For this review, take the finished solid that the model builds, in its own axes (mm). A direction names the side the tool comes from. Give positions to 0.01 mm unless a question says otherwise; leave off trailing zeros. Loops run counter-clockwise (first coordinate to the right, second up) from the corner with the lowest first, then second, coordinate; pieces in that order, holes last.
```python
from build123d import *

# Parameters (mm, degrees)
SKETCH1_W                  = 12.065
SKETCH1_H                  = 15.875
BASE_DEPTH                 = 15.875
SKETCH3_R                  = 1.397
SHAFTHOLE_DEPTH            = 19.745948562
SKETCH7_W                  = 18.144441676
SKETCH7_H                  = 22.667604572
SKETCH7_W_2                = 6.35
SKETCH7_H_2                = 10.16
CUT_EXTRUDE1_DEPTH         = 10.795
F_4_40_TAPPED_HOLE1_REACH  = 27.692
F_4_40_TAPPED_HOLE1_BORE_R = 1.1303


with BuildPart() as part:
    # Sketch1 → Base (new body)
    with BuildSketch(Plane.XY):
        Rectangle(SKETCH1_W, SKETCH1_H)
    extrude(amount=BASE_DEPTH)

    # Sketch3 → ShaftHole (cut, through all)
    with BuildSketch(Plane(origin=(0, 0, 0), x_dir=(-1, 0, 0), z_dir=(0, 0, -1))):
        with Locations((0, 3.1877)):
            Circle(SKETCH3_R)
    extrude(amount=-SHAFTHOLE_DEPTH, mode=Mode.SUBTRACT)

    # Sketch7 → Cut-Extrude1 (cut)
    with BuildSketch(Plane(origin=(0, 7.9375, 0), x_dir=(1, 0, 0), z_dir=(0, 1, 0))):
        with Locations((0.669483701, -7.615912702)):
            Rectangle(SKETCH7_W, SKETCH7_H)
        with Locations((0, -5.08)):
            Rectangle(SKETCH7_W_2, SKETCH7_H_2, mode=Mode.SUBTRACT)
    extrude(amount=-CUT_EXTRUDE1_DEPTH, mode=Mode.SUBTRACT)

    # #4-40 Tapped Hole1 bore → #4-40 Tapped Hole1 (cut, up to next)
    with BuildSketch(Plane(origin=(5.103236707, 7.9375, -0.979692924), x_dir=(0, 0, 1), z_dir=(0, 1, 0)), mode=Mode.PRIVATE) as f_4_40_tapped_hole1_sk1:
        with Locations((6.059692924, -5.103236707)):
            Circle(F_4_40_TAPPED_HOLE1_BORE_R)
    f_4_40_tapped_hole1_tool1 = extrude(f_4_40_tapped_hole1_sk1.sketch, amount=-F_4_40_TAPPED_HOLE1_REACH, mode=Mode.PRIVATE) & part.part
    add(f_4_40_tapped_hole1_tool1.solids().sort_by_distance((0, 7.9375, 5.08))[0], mode=Mode.SUBTRACT)


solid = part.part
```
Item 1: Take a section at C-C on z = 5.08. Give the boundary of the cut face in (x, y) (1 decimal).
Answer:
outline: (-6, -7.9) - (6, -7.9) - (6, -2.9) - (3.2, -2.9) - (3.2, 7.9) - (1.1, 7.9) - (1.1, 4) arc R1.4 cw (long way) to (-1.1, 4) - (-1.1, 7.9) - (-3.2, 7.9) - (-3.2, -2.9) - (-6, -2.9) - close
Item 2: For L1, parallel to Z at x = 0, y = 6.9; L2, parallel to Y at x = 0, z = 7; L3, parallel to X at y = 5, z = 5.08 (3 decimals), list the stretches that pass through material, from the lowest coordinate up.
Answer:
L1: z = 0 to 3.95, 6.21 to 10.16
L2: y = -7.94 to 1.79, 4.58 to 7.94
L3: x = -3.175 to -1.13, 1.13 to 3.175
Item 3: Take a section at D-D on z = 8. Give the boundary of the cut face in (x, y) (1 decimal), and give its area (3 significant figures).
Answer:
outline: (-6, -7.9) - (6, -7.9) - (6, -2.9) - (3.2, -2.9) - (3.2, 7.9) - (-3.2, 7.9) - (-3.2, -2.9) - (-6, -2.9) - close; hole circle Ø2.8 at (0, 3.2)
area: 124 mm2
Item 4: Clearance check with flat-ended pins moving along their axes: pin 1 Ø7 at (x, y) = (-1, 0) entering from +Z (3 decimals); pin 2 Ø6 at (y, z) = (2.5, 2.5) entering from -X (3 decimals); pin 3 Ø8 at (y, z) = (4.5, 3.5) entering from +X (3 decimals). State where each tip first meets the part, or that it passes through.
Answer:
pin 1: stops at z = 15.875
pin 2: stops at x = -3.175
pin 3: stops at x = 3.175
Item 5: Tool access review of faces 5 (the flat face through (0, 1, 10.16)), 6 (the flat face through (3.175, 3, 5)), 7 (the flat face through (1, 7.938, 4)), 8 (the flat face through (-3.175, 3, 5)): name each direction out of +Z, -Z, +X, -X, +Y, -Y from which nothing blocks a thin tool from reaching the whole face with its end or side.
Answer:
face 5: +Z, +X, -X, +Y
face 6: +Z, -Z, +X, +Y
face 7: +Z, -Z, +X, -X, +Y
face 8: +Z, -Z, -X, +Y
Item 6: Take a section at B-B on x = 0. Give the boundary of the cut face in (y, z) (1 decimal), and give its area (3 significant figures).
Answer:
outline: (-7.9, 0) - (1.8, 0) - (1.8, 10.2) - (-2.9, 10.2) - (-2.9, 15.9) - (-7.9, 15.9) - close; (4.6, 0) - (7.9, 0) - (7.9, 3.9) - (4.6, 3.9) - close; (4.6, 6.2) - (7.9, 6.2) - (7.9, 10.2) - (4.6, 10.2) - close
area: 154 mm2
Item 7: Take a section at A-A on y = 3.5. Give the boundary of the cut face in (x, z) (3 decimals), and give its area (3 significant figures).
Answer:
outline: (-3.175, 0) - (-1.362, 0) - (-1.362, 10.16) - (-3.175, 10.16) - close; (1.362, 0) - (3.175, 0) - (3.175, 10.16) - (1.362, 10.16) - close
area: 36.8 mm2
Item 8: The part is to be moulded in two halves that separate along X. For faces 1 (the flat face through (-6.032, -5, 8)), 2 (the flat face through (0, -2, 0)), 3 (the cylindrical face through (0.34, 6, 6.16)), 4 (the cylindrical face through (0.303, 1.824, 5.009)), say which applies: released by +X, released by -X, zero draft, split by the parting line, or undercut.
Answer:
face 1: released by -X
face 2: zero draft
face 3: undercut
face 4: undercut
